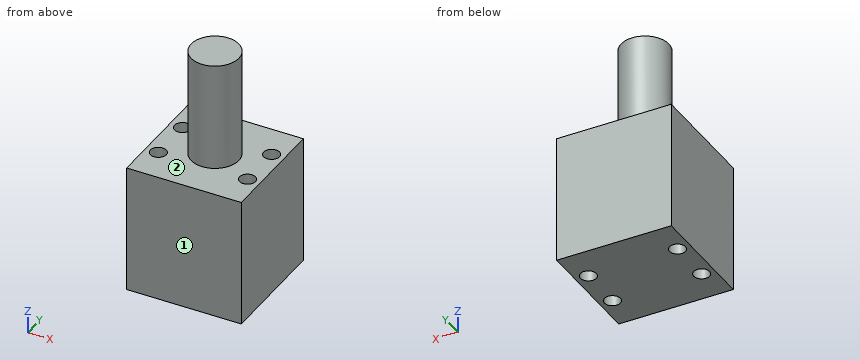
```python
from build123d import *

# Parameters (mm, degrees)
F0_R     = 7.5
F1_DEPTH = 74.4
F0_W     = 36
F0_H     = 36
F2_DEPTH = 40.4
F4_D     = 5


with BuildPart() as f1:
    # F0 (on Top) → F1 (new body)
    with BuildSketch(Plane.XY):
        Circle(F0_R)
    extrude(amount=F1_DEPTH)

    # F0 (on Top) → F2 (join)
    with BuildSketch(Plane.XY):
        Rectangle(F0_W, F0_H)
        Circle(F0_R, mode=Mode.SUBTRACT)
    extrude(amount=F2_DEPTH)

    # F4 (through all)
    with Locations(Plane(origin=(0, 0, 0), x_dir=(1, 0, 0), z_dir=(0, 0, -1))):
        with Locations((-14, 7), (14, 7), (14, -7), (-14, -7)):
            Hole(F4_D / 2)


solid = f1.part
```
For this review, take the finished solid that the model builds, in its own axes (mm). Face numbers are marked on the shaded views. A direction names the side the tool comes from. Round coordinates to 2 decimals unless told otherwise and drop trailing zeros. Loops run counter-clockwise (first coordinate to the right, second up) from the corner with the lowest first, then second, coordinate; pieces in that order, holes last.
(1) We need section A-A (x = 14). Give the boundary of the cut face in (y, z).
Returned:
outline: (-18, 0) - (-9.5, 0) - (-9.5, 40.4) - (-18, 40.4) - close; (-4.5, 0) - (4.5, 0) - (4.5, 40.4) - (-4.5, 40.4) - close; (9.5, 0) - (18, 0) - (18, 40.4) - (9.5, 40.4) - close
(2) Clearance check with flat-ended pins moving along their axes: P1, Ø3, axis at x = 14, y = -7, coming from the +Z side; P2, Ø3, axis at x = 9, y = -4.5, coming from the +Z side. State where each tip first meets the part, or that it passes through.
Returned:
P1: passes through
P2: stops at z = 40.4
(3) We need section B-B (y = -5.5). Give the boundary of the cut face in (x, z).
Returned:
outline: (-18, 0) - (-16, 0) - (-16, 40.4) - (-18, 40.4) - close; (-12, 0) - (12, 0) - (12, 40.4) - (5.1, 40.4) - (5.1, 74.4) - (-5.1, 74.4) - (-5.1, 40.4) - (-12, 40.4) - close; (16, 0) - (18, 0) - (18, 40.4) - (16, 40.4) - close
(4) Wall thickness on line 1 along Y through (x, z) = (14, 26); line 2 along Z through (x, y) = (11, 8); line 3 along Y through (x, z) = (13, 18.5): over which ranges is each line inside the solid? List them lowest first.
Returned:
line 1: y = -18 to -9.5, -4.5 to 4.5, 9.5 to 18
line 2: z = 0 to 40.4
line 3: y = -18 to -9.29, -4.71 to 4.71, 9.29 to 18
(5) Tool access review of the marked faces 1 and 2: name each direction out of +Z, -Z, +X, -X, +Y, -Y from which nothing blocks a thin tool from reaching the whole face with its end or side.
Returned:
face 1: +Z, -Z, +X, -X, -Y
face 2: +Z
(6) We need section C-C (y = 0). Give the boundary of the cut face in (x, z).
Returned:
outline: (-18, 0) - (18, 0) - (18, 40.4) - (7.5, 40.4) - (7.5, 74.4) - (-7.5, 74.4) - (-7.5, 40.4) - (-18, 40.4) - close
(7) We need section D-D (x = 3.5). Give the boundary of the cut face in (y, z).
Returned:
outline: (-18, 0) - (18, 0) - (18, 40.4) - (6.63, 40.4) - (6.63, 74.4) - (-6.63, 74.4) - (-6.63, 40.4) - (-18, 40.4) - close
